Read the model definition and answer for the solid it produces. Units are mm, in the model's axes. Give positions to 0.01 mm unless a question says otherwise; leave off trailing zeros. Loops run counter-clockwise (first coordinate to the right, second up) from the corner with the lowest first, then second, coordinate; pieces in that order, holes last. Notation, with made-up numbers: (2, 39) -> (7, 39) arc R21 ccw to (7, 53) -> close; hole circle Ø3 at (31.5, -34.5). An arc over 180 degrees is marked (long way). Answer as CSV lines item,"result". Start each with the question number.
```python
from build123d import *

# Parameters (mm, degrees)
F1_DEPTH = 2
F0_W     = 53
F0_H     = 9
F0_H_2   = 10
F0_W_2   = 6
F0_H_3   = 1
F2_DEPTH = 1
F3_DEPTH = 0.5
F4_DEPTH = 2


with BuildPart() as f1:
    # F0 (on Top) → F1 (new body)
    with BuildSketch(Plane.XY):
        Polygon((56.5, -30), (60, -30), (60, 30), (-60, 30), (-60, -30), (-56.5, -30), (-56.5, -20), (-56.5, -19), (-56.5, -10), (-56.5, -9), (-56.5, 0), (-56.5, 1), (-56.5, 10), (-56.5, 11), (-56.5, 20), (-3.5, 20), (-3.5, 11), (-3.5, 10), (-3.5, 1), (-3.5, 0), (-3.5, -9), (-3.5, -10), (-3.5, -19), (-3.5, -20), (-3.5, -30), (3.5, -30), (3.5, -20), (3.5, -19), (3.5, -10), (3.5, -9), (3.5, 0), (3.5, 1), (3.5, 10), (3.5, 11), (3.5, 20), (56.5, 20), (56.5, 11), (56.5, 10), (56.5, 1), (56.5, 0), (56.5, -9), (56.5, -10), (56.5, -19), (56.5, -20), align=None)
    extrude(amount=F1_DEPTH)

    # F0 (on Top) → F2 (join)
    with BuildSketch(Plane.XY):
        with Locations((-30, 15.5)):
            Rectangle(F0_W, F0_H)
        with Locations((-30, 5.5)):
            Rectangle(F0_W, F0_H)
        with Locations((-30, -4.5)):
            Rectangle(F0_W, F0_H)
        with Locations((-30, -14.5)):
            Rectangle(F0_W, F0_H)
        with Locations((-30, -25)):
            Rectangle(F0_W, F0_H_2)
        with Locations((-30, -25.271689)):
            Rectangle(F0_W_2, F0_H_3, mode=Mode.SUBTRACT)
        with Locations((30, -25)):
            Rectangle(F0_W, F0_H_2)
        with Locations((30, -25.271689)):
            Rectangle(F0_W_2, F0_H_3, mode=Mode.SUBTRACT)
        with Locations((30, -14.5)):
            Rectangle(F0_W, F0_H)
        with Locations((30, -4.5)):
            Rectangle(F0_W, F0_H)
        with Locations((30, 5.5)):
            Rectangle(F0_W, F0_H)
        with Locations((30, 15.5)):
            Rectangle(F0_W, F0_H)
    extrude(amount=F2_DEPTH)

    # F0 (on Top) → F3 (join)
    with BuildSketch(Plane.XY):
        with Locations((-30, 10.5)):
            Rectangle(F0_W, F0_H_3)
        with Locations((-30, 0.5)):
            Rectangle(F0_W, F0_H_3)
        with Locations((-30, -9.5)):
            Rectangle(F0_W, F0_H_3)
        with Locations((-30, -19.5)):
            Rectangle(F0_W, F0_H_3)
        with Locations((30, -19.5)):
            Rectangle(F0_W, F0_H_3)
        with Locations((30, -9.5)):
            Rectangle(F0_W, F0_H_3)
        with Locations((30, 0.5)):
            Rectangle(F0_W, F0_H_3)
        with Locations((30, 10.5)):
            Rectangle(F0_W, F0_H_3)
    extrude(amount=F3_DEPTH)

    # F0 (on Top) → F4 (join)
    with BuildSketch(Plane.XY):
        with Locations((-30, -25.271689)):
            Rectangle(F0_W_2, F0_H_3)
        with Locations((30, -25.271689)):
            Rectangle(F0_W_2, F0_H_3)
    extrude(amount=F4_DEPTH)


solid = f1.part
```
(1) Find section A-A on z = 1.7. Write down the section's boundary in (x, y), then the cut area to 3 significant figures.
(2) Find section B-B on x = -22. Write down the section's boundary in (y, z).
(3) Find the intervals of material crossed by line 1 along X through (y, z) = (-3, 1.2); line 2 along Y through (x, z) = (29.5, 0.65); line 3 along Z through (x, y) = (-12.5, 6.5), in increasing order. Write a range as from..to.
(4) Each of these flat-tipped pins is pushed along its axis until it touches: P1, Ø7, axis at x = -20.5, y = 5, coming from the +Z side; P2, Ø0.5, axis at x = -24, y = -9.5, coming from the +Z side. Where does it stop, or does it pass through?
(5) Find section C-C on y = -17.5. Write down the section's boundary in (x, z), then the cut area to 3 significant figures.
(6) The mould has two halves that part along X. Classify faces 1 (the face through (30, 16, 1)), 2 (the face through (0, 16, 2)): pulls with the +X half, pulls with the -X half, needs draft (parallel to the pull), parting line crosses it, or undercut.
Answer block:
1,outline,"(-60, -30) -> (-56.5, -30) -> (-56.5, 20) -> (-3.5, 20) -> (-3.5, -30) -> (3.5, -30) -> (3.5, 20) -> (56.5, 20) -> (56.5, -30) -> (60, -30) -> (60, 30) -> (-60, 30) -> close; (-33, -25.77) -> (-27, -25.77) -> (-27, -24.77) -> (-33, -24.77) -> close; (27, -25.77) -> (33, -25.77) -> (33, -24.77) -> (27, -24.77) -> close"
1,area,"1,910 mm2"
2,outline,"(-30, 0) -> (30, 0) -> (30, 2) -> (20, 2) -> (20, 1) -> (11, 1) -> (11, 0.5) -> (10, 0.5) -> (10, 1) -> (1, 1) -> (1, 0.5) -> (0, 0.5) -> (0, 1) -> (-9, 1) -> (-9, 0.5) -> (-10, 0.5) -> (-10, 1) -> (-19, 1) -> (-19, 0.5) -> (-20, 0.5) -> (-20, 1) -> (-30, 1) -> close"
3,line 1,"x = -60..-56.5, -3.5..3.5, 56.5..60"
3,line 2,"y = -30..-20, -19..-10, -9..0, 1..10, 11..30"
3,line 3,"z = 0..1"
4,P1,"stops at z = 1"
4,P2,"stops at z = 0.5"
5,outline,"(-60, 0) -> (60, 0) -> (60, 2) -> (56.5, 2) -> (56.5, 1) -> (3.5, 1) -> (3.5, 2) -> (-3.5, 2) -> (-3.5, 1) -> (-56.5, 1) -> (-56.5, 2) -> (-60, 2) -> close"
5,area,"134 mm2"
6,face 1,"undercut"
6,face 2,"needs draft"
